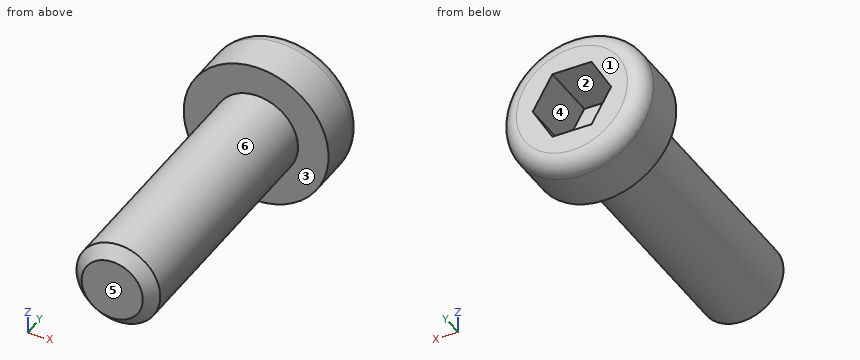
```python
from build123d import *

# Parameters (mm, degrees)
SKETCH1_R           = 3.2
BOSS_EXTRUDE1_DEPTH = 2.6
FILLET1_R           = 0.75
SKETCH2_R           = 1.85
BOSS_EXTRUDE2_DEPTH = 11.7
CHAMFER1_SIZE       = 0.5


with BuildPart() as part:
    # Sketch1 → Boss-Extrude1 (new body)
    with BuildSketch(Plane(origin=(0, 0, 0), x_dir=(1, 0, 0), z_dir=(0, 1, 0))):
        with Locations(Location((0, 0, 0), (0, 0, 270))):
            Circle(SKETCH1_R)
        Polygon((1.732050808, 0), (0.866025404, 1.5), (-0.866025404, 1.5), (-1.732050808, 0), (-0.866025404, -1.5), (0.866025404, -1.5), align=None, mode=Mode.SUBTRACT)
    extrude(amount=BOSS_EXTRUDE1_DEPTH)

    # Fillet1
    fillet1_edges = [part.edges().sort_by_distance(p)[0] for p in [
        (0, 2.6, -3.2),
    ]]
    fillet(fillet1_edges, radius=FILLET1_R)

    # Sketch2 → Boss-Extrude2 (add)
    with BuildSketch(Plane.XZ):
        with Locations(Location((0, 0, 0), (0, 0, 90))):
            Circle(SKETCH2_R)
    extrude(amount=BOSS_EXTRUDE2_DEPTH)

    # Chamfer1
    chamfer1_edges = [part.edges().sort_by_distance(p)[0] for p in [
        (0, -11.7, -1.85),
    ]]
    chamfer(chamfer1_edges, length=CHAMFER1_SIZE)


solid = part.part
```
Geometry: final body of the model. Coordinates: model frame, mm. Face numbers are marked on the shaded views. A direction names the side the tool comes from. Coordinates: 2 decimals unless noted, no trailing zeros. Write each loop counter-clockwise with the first axis right and the second up, starting at its lowest first coordinate (ties: lowest second). Pieces come first, ordered by that corner, then holes. Notation, with made-up numbers: M 32,-9 L 57,-9 A15 ccw 57,3 Z; hole C -7,85 d9. An arc over 180 degrees is marked long. Answer as CSV lines item,"result". Start each with the question number.
Q1. Cut plane B-B on y = -0.5. Return the cut outline in (x, z).
Q2. Pin query (flat end, axial travel): P1, Ø1, axis at y = -9.5, z = 1.5, coming from the +X side; P2, Ø3, axis at x = -2.5, y = -4.5, coming from the -Z side; P3, Ø3, axis at x = 0.5, y = -3, coming from the -Z side. Return the tip coordinate at first contact, or that it passes through.
Q3. Cut plane A-A on x = 0. Return the cut outline in (y, z), then the cut area to 3 significant figures.
Q4. Mould query, pull axis X, two halves, no side actions, for the marked faces 4, 5 and 6. Classes: released by +X, released by -X, zero draft, split by the parting line, or undercut.
Q5. Line query: line 1 (Y direction, x = -2.5, z = 0); line 2 (Z direction, x = 0.5, y = 1.5); line 3 (Y direction, x = 0.75, z = 0.5). Output: solid intervals per line, ascending. Write a range as from..to.
Q6. Reachability of the marked faces 1, 2 and 3 from +Z, -Z, +X, -X, +Y, -Y: full face, straight path, thin tool, end or side. Return the list, or none.
Findings below:
1,outline,"C 0,0 d3.7"
2,P1,"stops at x = 1.56"
2,P2,"stops at z = -1.56"
2,P3,"stops at z = -1.85"
3,outline,"M -11.7,-1.35 L -11.2,-1.85 L 0,-1.85 L 0,-3.2 L 1.85,-3.2 A0.75 ccw 2.6,-2.45 L 2.6,-1.5 L 0,-1.5 L 0,1.5 L 2.6,1.5 L 2.6,2.45 A0.75 ccw 1.85,3.2 L 0,3.2 L 0,1.85 L -11.2,1.85 L -11.7,1.35 Z"
3,area,"51.6 mm2"
4,face 4,"undercut"
4,face 5,"zero draft"
4,face 6,"split by the parting line"
5,line 1,"y = 0..2.6"
5,line 2,"z = -3.16..-1.5, 1.5..3.16"
5,line 3,"y = -11.7..0"
6,face 1,"+Z, -Z, +X, -X, +Y"
6,face 2,"+Y"
6,face 3,"-Y"
